```python
from build123d import *

# Parameters (mm, degrees)
BOSS_EXTRUDE1_DEPTH = 10.5
BOSS_EXTRUDE2_START = -10.5
BOSS_EXTRUDE2_DEPTH = 10.5
SKETCH3_R           = 1.375
CUT_EXTRUDE1_DEPTH  = 70.224771272


with BuildPart() as part:
    # Sketch1 → Boss-Extrude1 (new body)
    with BuildSketch(Plane(origin=(0, 0, 0), x_dir=(0, 0, -1), z_dir=(1, 0, 0))):
        with BuildLine():
            Line((27, 10), (5, 10))
            ThreePointArc((5, 10), (0, 5), (5, 0))
            Line((5, 0), (27, 0))
            ThreePointArc((27, 0), (32, 5), (27, 10))
        make_face()
    extrude(amount=BOSS_EXTRUDE1_DEPTH)

    # Sketch2 → Boss-Extrude2 (add)
    with BuildSketch(Plane(origin=(10.5, 0, 0), x_dir=(0, 0, -1), z_dir=(1, 0, 0)).offset(BOSS_EXTRUDE2_START)):
        with BuildLine():
            add(Edge.make_bspline(
                [(63.752972286, 17.872423117), (45.928882678, 26.563787963), (31.059268621, 10), (13.694974759, 10)],
                knots=[0, 0, 0, 0, 1, 1, 1, 1], degree=3))
            Line((13.694974759, 10), (27, 10))
            ThreePointArc((27, 10), (31.87285141, 6.120410255), (29.183837075, 0.502127655))
            Line((29.183837075, 0.502127655), (38.08542066, 4.824084077))
            add(Edge.make_bspline(
                [(38.08542066, 4.824084077), (46.797509509, 11.895222457), (57.948000409, 11.067843667)],
                knots=[0, 0, 0, 1, 1, 1], degree=2))
            Line((57.948000409, 11.067843667), (65.313809691, 14.189518476))
            Line((65.313809691, 14.189518476), (63.752972286, 17.872423117))
        make_face()
    extrude(amount=BOSS_EXTRUDE2_DEPTH)

    # Sketch3 → Cut-Extrude1 (cut, through all)
    with BuildSketch(Plane(origin=(10.5, 0, 0), x_dir=(0, 0, -1), z_dir=(1, 0, 0))):
        with Locations((5, 5)):
            Circle(SKETCH3_R)
        with Locations((27, 5)):
            Circle(SKETCH3_R)
    extrude(amount=-CUT_EXTRUDE1_DEPTH, mode=Mode.SUBTRACT)


solid = part.part
```
Build history of the part. All positions in model axes, mm. Round coordinates to 2 decimals unless told otherwise and drop trailing zeros. Loops run counter-clockwise (first coordinate to the right, second up) from the corner with the lowest first, then second, coordinate; pieces in that order, holes last.
Item 1: Pin check, flat tips, straight feed: P1, Ø3, axis at x = 8.5, z = -16, coming from the +Y side; P2, Ø2, axis at y = 5, z = -5, coming from the +X side; P3, Ø6, axis at x = 1.5, y = 4, coming from the -Z side; P4, Ø2, axis at x = 1.5, y = 17.5, coming from the -Z side. Stop position of each tip, or through.
Item 2: Two-plate mould, pull along Z, no slides. Class faces 1 (the face through (5, 10, -9)), 2 (the face through (5.324, 5.06, -25.626)), 3 (the face through (5.176, 16.005, -64.544)): released by +Z, released by -Z, zero draft, split by the parting line, or undercut.
Item 3: Drill centre lines: line 1 along Y through (x, z) = (4, -5) (3 decimals); line 2 along Z through (x, y) = (1.5, 4.5); line 3 along Z through (x, y) = (3.25, 4.75). Where is each one in solid material? Low to high.
Item 4: Saw through at B-B (x = 8.5). State how many separate pieces and enclosed holes the cut face has, then the cut area to 3 significant figures.
Item 5: Saw through at A-A (y = 4.25). List the corners of the cut face in (x, z).
Worked answers:
1. P1: stops at y = 10.25
1. P2: passes through
1. P3: stops at z = -41.12
1. P4: stops at z = -64.33
2. face 1: zero draft
2. face 2: undercut
2. face 3: released by -Z
3. line 1: y = 0 to 3.625, 6.375 to 10
3. line 2: z = -37.42 to -28.28, -25.72 to -6.28, -3.72 to -0.03
3. line 3: z = -37.93 to -28.35, -25.65 to -6.35, -3.65 to -0.01
4. separate pieces: 1
4. enclosed holes: 2
4. area: 642 mm2
5. outline: (0, -36.9) - (10.5, -36.9) - (10.5, -28.15) - (0, -28.15) - close; (0, -25.85) - (10.5, -25.85) - (10.5, -6.15) - (0, -6.15) - close; (0, -3.85) - (10.5, -3.85) - (10.5, -0.06) - (0, -0.06) - close
